For this review, take the finished solid that the model builds, in its own axes (mm). A direction names the side the tool comes from. Round coordinates to 2 decimals unless told otherwise and drop trailing zeros. Order: outer loops, then holes, each group sorted by start corner. A loop starts at its lowest first (then second) coordinate and runs counter-clockwise, first axis right, second up. Notation, with made-up numbers: M 2.25,80 L 31.25,80 A29 ccw 31.25,117 Z; hole C -19.5,45.25 d1. An arc over 180 degrees is marked long. Use a Markdown table: item, result.
from build123d import *

# Parameters (mm, degrees)
F1_DEPTH   = 685.8
F2_R       = 5.08
F3_W       = 38.1
F3_H       = 38.1
F1_FACE1_W = 1361.44
F1_FACE1_H = 608.8846015944
F4_DEPTH   = 76.201


with BuildPart() as f1:
    # F0 (on Right) → F1 (new body, symmetric)
    with BuildSketch(Plane.YZ):
        Polygon((927.1, 47.7274174528), (76.2, 47.7274174528), (76.2, 514.3720190472), (0, 514.3720190472), (0, -104.6725825472), (76.2, -104.6725825472), (927.1, -104.6725825472), align=None)
    extrude(amount=F1_DEPTH, both=True)

    # F2
    f2_edges = [f1.edges().sort_by_distance(p)[0] for p in [
        (0, 76.2, 514.372019),
        (685.8, 76.2, 281.049718),
        (-685.8, 76.2, 281.049718),
        (685.8, 501.65, 47.727417),
        (0, 927.1, 47.727417),
        (-685.8, 501.65, 47.727417),
        (0, 76.2, 47.727417),
        (685.8, 927.1, -28.472583),
        (-685.8, 927.1, -28.472583),
        (0, 927.1, -104.672583),
        (685.8, 463.55, -104.672583),
        (685.8, 0, 204.849718),
        (685.8, 38.1, 514.372019),
        (0, 0, 514.372019),
        (-685.8, 38.1, 514.372019),
        (-685.8, 0, 204.849718),
        (-685.8, 463.55, -104.672583),
        (0, 0, -104.672583),
    ]]
    fillet(f2_edges, radius=F2_R)

    # F3 (on face) + F1_face1 (on face) → F4 (cut, through all)
    with BuildSketch(Plane(origin=(0, 76.2, 0), x_dir=(-1, 0, 0), z_dir=(0, 1, 0))):
        with Locations((-555.6620976448, 401.3420190472)):
            Rectangle(F3_W, F3_H)
    with BuildSketch(Plane(origin=(0, 0, 204.84971825), x_dir=(1, 0, 0), z_dir=(0, -1, 0))):
        Rectangle(F1_FACE1_W, F1_FACE1_H)
    extrude(amount=-F4_DEPTH, dir=(0, 1, 0), mode=Mode.SUBTRACT)


solid = f1.part
Q1. Clearance check with flat-ended pins moving along their axes: pin 1 (8 mm diameter, centred on x = -468.5, z = 191, fed in from +Y); pin 2 (1 mm diameter, centred on x = -171.5, y = 434.5, fed in from +Z). State where each tip first meets the part, or that it passes through.
Determined:
| item | result |
|---|---|
| pin 1 | stops at y = 76.2 |
| pin 2 | stops at z = 47.73 |
Q2. Machinability: for faces 1 (the flat face through (556, 39, 382.292)), 2 (the flat face through (10, 76.2, 278)), 3 (the flat face through (10, 457, -104.673)), which of the approach directions +Z, -Z, +X, -X, +Y, -Y give a long, thin tool a straight path to every point of the face, cutting with its end or side? Answer none if there is none.
Determined:
| item | result |
|---|---|
| face 1 | +Y, -Y |
| face 2 | +Z, +X, -X, +Y |
| face 3 | -Z, +X, -X, +Y, -Y |
Q3. Add section C-C (x = 170.5). Write out the cut boundary in (y, z), then the cut area to 3 significant figures.
Determined:
| item | result |
|---|---|
| outline | M 0,-99.59 A5.08 ccw 5.08,-104.67 L 922.02,-104.67 A5.08 ccw 927.1,-99.59 L 927.1,42.65 A5.08 ccw 922.02,47.73 L 81.28,47.73 A5.08 cw 76.2,52.81 L 76.2,509.29 A5.08 ccw 71.12,514.37 L 5.08,514.37 A5.08 ccw 0,509.29 Z |
| area | 177,000 mm^2 |
Q4. Add section D-D (z = 265). Write out the cut boundary in (x, y), then the cut area to 3 significant figures.
Determined:
| item | result |
|---|---|
| outline | M -685.8,5.08 A5.08 ccw -680.72,0 L 680.72,0 A5.08 ccw 685.8,5.08 L 685.8,71.12 A5.08 ccw 680.72,76.2 L -680.72,76.2 A5.08 ccw -685.8,71.12 Z |
| area | 104,000 mm^2 |
Q5. Add section A-A (z = 401). Write out the cut boundary in (x, y).
Determined:
| item | result |
|---|---|
| outline | M -685.8,5.08 A5.08 ccw -680.72,0 L 536.61,0 L 536.61,76.2 L -680.72,76.2 A5.08 ccw -685.8,71.12 Z; M 574.71,0 L 680.72,0 A5.08 ccw 685.8,5.08 L 685.8,71.12 A5.08 ccw 680.72,76.2 L 574.71,76.2 Z |
Q6. Add section B-B (y = 689). Write out the cut boundary in (x, z), then the cut area to 3 significant figures.
Determined:
| item | result |
|---|---|
| outline | M -685.8,-99.59 A5.08 ccw -680.72,-104.67 L 680.72,-104.67 A5.08 ccw 685.8,-99.59 L 685.8,42.65 A5.08 ccw 680.72,47.73 L -680.72,47.73 A5.08 ccw -685.8,42.65 Z |
| area | 209,000 mm^2 |
Q7. Wall thickness on line 1 along Z through (x, y) = (367, 541); line 2 along Y through (x, z) = (69.5, 343.5); line 3 along Y through (x, z) = (-269, 50): over which ranges is each line inside the solid? List them lowest first. Write a range as [from, to].
Determined:
| item | result |
|---|---|
| line 1 | z = [-104.67, 47.73] |
| line 2 | y = [0, 76.2] |
| line 3 | y = [0, 77.05] |
Q8. Draft analysis for pull direction X (two halves, no side actions). For faces 4 (the flat face through (685.8, 360, 26)), 5 (the flat face through (556, 39, 420.392)), 6 (the flat face through (10, 927.1, -29)), state which applies: pulls with the +X half, pulls with the -X half, needs draft (parallel to the pull), parting line crosses it, or undercut.
Determined:
| item | result |
|---|---|
| face 4 | pulls with the +X half |
| face 5 | undercut |
| face 6 | needs draft |
